from build123d import *

# Parameters (mm, degrees)
F2_R     = 1.65
F3_DEPTH = 6.5
F4_SIZE  = 1.2
F5_R     = 1


# Not quite as in the source:
# - a feature names something its author has since deleted; it is built from what else it names


with BuildPart() as f1:
    # F0 (on Right) → F1 (revolve)
    with BuildSketch(Plane.YZ):
        Polygon((8.35, 0), (17.2, 0), (17.2, 6.5), (16.45, 6.5), (16.45, 2.9), (9.1, 2.9), (9.1, 6.5), (8.35, 6.5), align=None)
    revolve(axis=Axis((0, 0, -2.445915569), (0, 0, -1)))

    # F2 (on Top) → F3 (join, through all)
    with BuildSketch(Plane.XY):
        with BuildLine():
            Line((-12.9185614558, 11.3556492511), (-16.0443701425, 13.1603357378))
            ThreePointArc((-16.0443701425, 13.1603357378), (-20.6890755738, 11.8640180715), (-19.2967065825, 7.2471970193))
            Line((-19.2967065825, 7.2471970193), (-16.2926126828, 5.5127825977))
            ThreePointArc((-16.2926126828, 5.5127825977), (-14.8948966536, 8.6012820951), (-12.9185614558, 11.3556492511))
        make_face()
        with Locations((-17.7318701425, 10.2375)):
            Circle(F2_R, mode=Mode.SUBTRACT)
        with BuildLine():
            ThreePointArc((16.5081291827, 4.8292515868), (17.1346777754, 1.4976039307), (17.0955988557, -1.8922208557))
            Line((17.0955988557, -1.8922208557), (20.6912370752, -1.5776432733))
            ThreePointArc((20.6912370752, -1.5776432733), (23.752419757, 2.1483315823), (19.9637580849, 5.1315799411))
            Line((19.9637580849, 5.1315799411), (16.5081291827, 4.8292515868))
        make_face()
        with Locations((20.3970864434, 1.7845138328)):
            Circle(F2_R, mode=Mode.SUBTRACT)
    extrude(amount=F3_DEPTH)

    # F4
    f4_edges = [f1.edges().sort_by_distance(p)[0] for p in [
        (-19.38187, 10.2375, 0),
    ]]
    chamfer(f4_edges, length=F4_SIZE)

    # F5
    f5_edges = [f1.edges().sort_by_distance(p)[0] for p in [
        (0, -16.45, 2.9),
        (0, -9.1, 2.9),
    ]]
    fillet(f5_edges, radius=F5_R)


solid = f1.part
Source: CAD feature listing. Evaluate the final solid. Frame: model axes, mm. A direction names the side the tool comes from. Coordinates: 2 decimals unless noted, no trailing zeros. Loops run counter-clockwise (first coordinate to the right, second up) from the corner with the lowest first, then second, coordinate; pieces in that order, holes last. Notation, with made-up numbers: (44.5, 11.25) - (63.5, 11.25) arc R28 cw to (63.5, 40.25) - close; hole circle Ø7 at (70.25, 87). An arc over 180 degrees is marked (long way). One line per item, written item: value. Start each with the question number.
1. Contact query for flat-ended pins moving along their axis: P1, Ø1.5, axis at x = -3.5, y = -6.5, coming from the +Z side; P2, Ø1, axis at y = 5.5, z = 4, coming from the -X side; P3, Ø1.5, axis at x = -1, z = 3.5, coming from the -Y side; P4, Ø1, axis at x = 9, z = 1.5, coming from the +Y side. Output: stop coordinate, or through.
2. Section A-A (x = 0). Return the cut outline in (y, z), and give its area (3 significant figures).
3. Set-up query: faces 4 (the flat face through (-14.46, 12.245, 3.204)), 5 (the cylindrical face through (-20.65, 11.93, 3.2)), 6 (the cylindrical face through (-16.059, -3.566, 5.182)), 7 (the flat face through (-3, 8, 6.5)), 8 (the flat face through (-17.816, 6.392, 3.204)). Return all of +Z, -Z, +X, -X, +Y, -Y with unobstructed straight access to the full face (end or side cutting, diameter ignored); none if empty.
4. Mould query, pull axis X, two halves, no side actions, for faces 1 (the flat face through (7, -7, 0)), 2 (the flat face through (18.868, -1.737, 3.204)), 3 (the cylindrical face through (2.508, 7.964, 3.204)). Classes: pulls with the +X half, pulls with the -X half, needs draft (parallel to the pull), parting line crosses it, or undercut.
5. Section B-B (z = 5.5). State how many separate pieces and enclosed holes the cut face has, and give its area (3 significant figures).
6. Ray query, L1, parallel to X at y = -1, z = 4; L2, parallel to X at y = 1, z = 6; L3, parallel to X at y = -6, z = 5. Return the intervals inside material, ascending.
Verdict:
1. P1: passes through
1. P2: stops at x = -17.14
1. P3: stops at y = -17.2
1. P4: stops at y = 14.95
2. outline: (-17.2, 0) - (-8.35, 0) - (-8.35, 6.5) - (-9.1, 6.5) - (-9.1, 3.9) arc R1 cw to (-10.1, 2.9) - (-15.45, 2.9) arc R1 cw to (-16.45, 3.9) - (-16.45, 6.5) - (-17.2, 6.5) - close; (8.35, 0) - (17.2, 0) - (17.2, 6.5) - (16.45, 6.5) - (16.45, 3.9) arc R1 cw to (15.45, 2.9) - (10.1, 2.9) arc R1 cw to (9.1, 3.9) - (9.1, 6.5) - (8.35, 6.5) - close
2. area: 63.0 mm2
3. face 4: +Z, -Z, +Y
3. face 5: +Z, -Z
3. face 6: +Z
3. face 7: +Z, +X, -X, +Y, -Y
3. face 8: +Z, -Z, -X
4. face 1: needs draft
4. face 2: pulls with the +X half
4. face 3: undercut
5. separate pieces: 2
5. enclosed holes: 4
5. area: 185 mm2
6. L1: x = -17.17 to -16.42, -9.04 to -8.29, 8.29 to 9.04, 16.42 to 22.3
6. L2: x = -17.17 to -16.42, -9.04 to -8.29, 8.29 to 9.04, 16.42 to 18.95, 21.85 to 23.68
6. L3: x = -16.12 to -15.32, -6.84 to -5.81, 5.81 to 6.84, 15.32 to 16.12
